Answer from the drawing. Dimensions are ordinates in mm from the lowest x, y and z of the part. A direction names the side the tool comes from. Give positions to 0.01 mm unless a question says otherwise; leave off trailing zeros. Loops run counter-clockwise (first coordinate to the right, second up) from the corner with the lowest first, then second, coordinate; pieces in that order, holes last.
Item 1: A tool of negligible diameter and unlimited length cuts with its end or side. For the marked faces 1, 2 and 3, from which of +Z, -Z, +X, -X, +Y, -Y can it reach the whole face along a straight path? Write none if from no direction.
Item 2: Consider line 1 along Z through (x, y) = (9, 1) (1 decimal); line 2 along X through (y, z) = (4.75, 3); line 3 along Z through (x, y) = (7.5, 11.5). Determine where each line is inside the solid, lowest interval first.
Item 3: Section A-A, the plane z = 3 is taken. Give the vertices of the cut face in (x, y).
Item 4: Section C-C, the plane x = 3.5 is taken. Give the vertices of the cut face in (y, z).
Item 5: This flat-tipped pin is pushed along its axis until it touches: pin 1 Ø3 at (x, z) = (7.5, 3) entering from -Y. Where does it stop, or does it pass through?
Item 6: Section B-B, the plane y = 16.75 is taken. Give the vertices of the cut face in (x, z).
Item 7: Section D-D, the plane y = 6 is taken. Give the vertices of the cut face in (x, z), and give its area (3 significant figures).
Item 8: The mould has two halves that part along Z. Classify the marked faces 4, 5, 6 and 7: pulls with the +Z half, pulls with the -Z half, needs draft (parallel to the pull), parting line crosses it, or undercut.
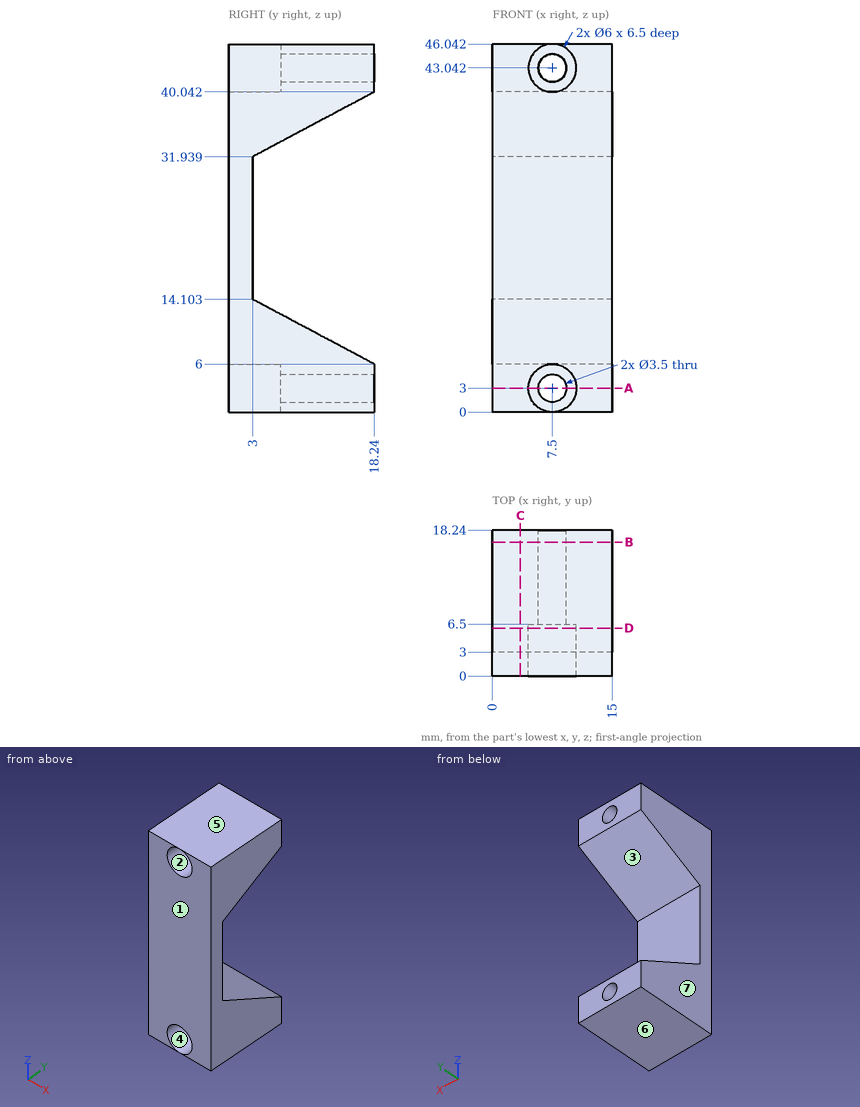
Worked answers:
1. face 1: +Z, -Z, +X, -X, -Y
1. face 2: -Y
1. face 3: +X, -X, +Y
2. line 1: z = 0 to 0.4, 5.6 to 40.4, 45.6 to 46
2. line 2: x = 0 to 4.5, 10.5 to 15
2. line 3: z = 0 to 1.25, 4.75 to 9.58, 36.46 to 41.29, 44.79 to 46.04
3. outline: (0, 0) - (4.5, 0) - (4.5, 6.5) - (5.75, 6.5) - (5.75, 18.24) - (0, 18.24) - close; (9.25, 6.5) - (10.5, 6.5) - (10.5, 0) - (15, 0) - (15, 18.24) - (9.25, 18.24) - close
4. outline: (0, 0) - (18.24, 0) - (18.24, 6) - (3, 14.1) - (3, 31.94) - (18.24, 40.04) - (18.24, 46.04) - (0, 46.04) - close
5. pin 1: passes through
6. outline: (0, 0) - (15, 0) - (15, 6.79) - (0, 6.79) - close; (0, 39.25) - (15, 39.25) - (15, 46.04) - (0, 46.04) - close; hole circle Ø3.5 at (7.5, 3); hole circle Ø3.5 at (7.5, 43.04)
7. outline: (0, 0) - (15, 0) - (15, 12.51) - (0, 12.51) - close; (0, 33.53) - (15, 33.53) - (15, 46.04) - (0, 46.04) - close; hole circle Ø6 at (7.5, 3); hole circle Ø6 at (7.5, 43.04)
7. area: 319 mm2
8. face 4: undercut
8. face 5: pulls with the +Z half
8. face 6: pulls with the -Z half
8. face 7: needs draft
